CAD build for the part. Positions are in the model's coordinates, mm. A direction names the side the tool comes from. Round coordinates to 2 decimals unless told otherwise and drop trailing zeros. Order: outer loops, then holes, each group sorted by start corner. A loop starts at its lowest first (then second) coordinate and runs counter-clockwise, first axis right, second up. Notation, with made-up numbers: M 16,34 L 42,34 A12 cw 42,43 Z; hole C -0.75,26.25 d6. An arc over 180 degrees is marked long. Answer as a JSON object with one key per item and string values.
```python
from build123d import *

# Parameters (mm, degrees)
BOSS_EXTRUDE1_DEPTH = 20
CUT_EXTRUDE1_REACH  = 90.171
SKETCH2_R           = 2.05
SKETCH3_W           = 20
SKETCH3_H           = 5.2
CUT_EXTRUDE2_DEPTH  = 16
SKETCH4_R           = 2.55
CUT_EXTRUDE3_DEPTH  = 97.113982306


with BuildPart() as part:
    # Sketch1 → Boss-Extrude1 (new body)
    with BuildSketch(Plane.XY):
        with BuildLine():
            ThreePointArc((0, -45), (-45, 0), (0, 45))
            Line((0, 45), (0, 60))
            Line((0, 60), (-4, 60))
            Line((-4, 60), (-4, 49.839743178))
            ThreePointArc((-4, 49.839743178), (-34.087674646, 36.579098366), (-49.434299833, 7.5))
            Line((-49.434299833, 7.5), (-65.434299833, 7.5))
            Line((-65.434299833, 7.5), (-65.434299833, -7.5))
            Line((-65.434299833, -7.5), (-49.434299833, -7.5))
            ThreePointArc((-49.434299833, -7.5), (-34.087674646, -36.579098366), (-4, -49.839743178))
            Line((-4, -49.839743178), (-4, -60))
            Line((-4, -60), (0, -60))
            Line((0, -60), (0, -45))
        make_face()
    extrude(amount=BOSS_EXTRUDE1_DEPTH)

    # Sketch2 → Cut-Extrude1 (cut, up to next)
    with BuildSketch(Plane.ZY.offset(4), mode=Mode.PRIVATE) as cut_extrude1_sk1:
        with Locations(Location((10, 55, 0), (0, 0, 270))):
            Circle(SKETCH2_R)
    cut_extrude1_tool1 = extrude(cut_extrude1_sk1.sketch, amount=-CUT_EXTRUDE1_REACH, mode=Mode.PRIVATE) & part.part
    cut_extrude1 = cut_extrude1_tool1.solids().sort_by_distance((-4, 55, 10))[0]
    add(cut_extrude1, mode=Mode.SUBTRACT)

    # Mirror1: Cut-Extrude1 across plane
    add(cut_extrude1.mirror(Plane.ZX), mode=Mode.SUBTRACT)

    # Sketch3 → Cut-Extrude2 (cut)
    with BuildSketch(Plane.ZY.offset(65.434299833)):
        with Locations((10, 0)):
            Rectangle(SKETCH3_W, SKETCH3_H)
    extrude(amount=-CUT_EXTRUDE2_DEPTH, mode=Mode.SUBTRACT)

    # Sketch4 → Cut-Extrude3 (cut, through all)
    with BuildSketch(Plane(origin=(0, 7.5, 0), x_dir=(1, 0, 0), z_dir=(0, 1, 0))):
        with Locations(Location((-57.434299833, -10, 0), (0, 0, 90))):
            Circle(SKETCH4_R)
    extrude(amount=-CUT_EXTRUDE3_DEPTH, mode=Mode.SUBTRACT)


solid = part.part
```
Item 1: Wall check: line 1 along Y through (x, z) = (-62, 13.75); line 2 along Y through (x, z) = (-25, 3.25); line 3 along X through (y, z) = (50, 3). Give the ranges that are in metal, low to high. Write a range as [from, to].
Worked answers:
{"line 1": "y = [-7.5, -2.6], [2.6, 7.5]", "line 2": "y = [-43.3, -37.42], [37.42, 43.3]", "line 3": "x = [-4, 0]"}
Item 2: Saw through at A-A on z = 10. State how many separate pieces and enclosed holes the cut face has, and give its area (3 significant figures).
Worked answers:
{"separate pieces": "5", "enclosed holes": "0", "area": "895 mm2"}
Item 3: 3-axis set-ups, long thin cutter, end or side, ignore diameter. For faces 4 (the flat face through (-55.5, 7.5, 7.6)), 5 (the flat face through (-4, -54.8, 7.6)), 6 (the flat face through (-59.3, -2.6, 12.1)): which of +Z, -Z, +X, -X, +Y, -Y reach the whole face in a straight line?
Worked answers:
{"face 4": "+Z, -Z, -X, +Y", "face 5": "+Z, -Z, -X, -Y", "face 6": "+Z, -Z, -X"}
Item 4: Saw through at B-B on y = 55. List the corners of the cut face in (x, z), and give its area (3 significant figures).
Worked answers:
{"outline": "M -4,0 L 0,0 L 0,7.95 L -4,7.95 Z; M -4,12.05 L 0,12.05 L 0,20 L -4,20 Z", "area": "63.6 mm2"}
Item 5: Saw through at C-C on x = -56. List the corners of the cut face in (y, z), and give its area (3 significant figures).
Worked answers:
{"outline": "M -7.5,0 L -2.6,0 L -2.6,7.89 L -7.5,7.89 Z; M -7.5,12.11 L -2.6,12.11 L -2.6,20 L -7.5,20 Z; M 2.6,0 L 7.5,0 L 7.5,7.89 L 2.6,7.89 Z; M 2.6,12.11 L 7.5,12.11 L 7.5,20 L 2.6,20 Z", "area": "155 mm2"}
Item 6: Drop flat-ended pins along their axis: pin 1 Ø3 at (y, z) = (17.5, 8) entering from -X; pin 2 Ø1 at (y, z) = (11.5, 15) entering from +X; pin 3 Ø8 at (x, z) = (-53.5, 8) entering from +Y; pin 4 Ø2 at (x, y) = (-27, -37) entering from -Z. Give the stop position or say it passes through.
Worked answers:
{"pin 1": "stops at x = -47.37", "pin 2": "stops at x = -43.37", "pin 3": "stops at y = 7.5", "pin 4": "stops at z = 0"}
Item 7: Saw through at D-D on x = -35.5. List the corners of the cut face in (y, z), and give its area (3 significant figures).
Worked answers:
{"outline": "M -35.21,0 L -27.65,0 L -27.65,20 L -35.21,20 Z; M 27.65,0 L 35.21,0 L 35.21,20 L 27.65,20 Z", "area": "302 mm2"}
Item 8: Two-plate mould, pull along Z, no slides. Class faces 1 (the flat face through (-45, -4, 20)), 2 (the cylindrical face through (-59.963, 5.084, 10.332)), 3 (the flat face through (-59.3, 2.6, 12.1)): released by +Z, released by -Z, zero draft, split by the parting line, or undercut.
Worked answers:
{"face 1": "released by +Z", "face 2": "undercut", "face 3": "zero draft"}
